Autodesk Inventor part; units mm, degrees
ref_plane "YZ Plane" through (0, 0, 0) normal (1, 0, 0) x (0, 1, 0)
ref_plane "XZ Plane" through (0, 0, 0) normal (0, 1, 0) x (-1, 0, 0)
ref_plane "XY Plane" through (0, 0, 0) normal (0, 0, 1) x (1, 0, 0)
sketch "Boceto2" plane through (0, 0, 0) normal (0, 0, 1) x (1, 0, 0)
  line L0 (-105.6698, 187.1112) -> (110.1141, 187.1112) construction
  line L1 (110.1141, 187.1112) -> (110.1141, -25.0762) construction
  line L2 (110.1141, -25.0762) -> (-105.6698, -25.0762) construction
  line L3 (-105.6698, -25.0762) -> (-105.6698, 187.1112) construction
  line L4 (0, 0) -> (0, 52.867)
  line L5 (0, 52.867) -> (0, 0)
  line L6 (-43.8447, 1.5105) -> (-43.8447, 13.5944)
  line L7 (-43.8447, 13.5944) -> (-37.8028, 21.1468)
  line L8 (-37.8028, 21.1468) -> (-39.3133, 27.944)
  line L9 (-39.3133, 27.944) -> (-36.2923, 36.2517)
  line L10 (-36.2923, 36.2517) -> (-32.6671, 40.7831)
  line L11 (-32.6671, 40.7831) -> (-30.2503, 43.8041)
  line L12 (-30.2503, 43.8041) -> (-27.2294, 47.5803)
  line L13 (-27.2294, 47.5803) -> (-27.2294, 52.867)
  line L14 (-27.2294, 52.867) -> (-23, 52.867)
  line L15 (0, 52.867) -> (-23, 52.867)
  line L16 (-27.2294, 52.867) -> (-23, 52.867)
  line L17 (0, 0) -> (-43.8447, 0)
  line L18 (-43.8447, 0) -> (-43.8447, 1.5105)
  dimension "d18" = 23
revolve "Revolución1" add sketch "Boceto2" angle 360 about axis through (0, 0, 0) along (0, 1, 0)
properties part number "KINGHT BASE 1.1"
Can you work these out from the model? Positions are in its coordinate system, mm. A direction names the side the tool comes from. Give positions to 0.01 mm unless a question says otherwise; leave off trailing zeros. Loops run counter-clockwise (first coordinate to the right, second up) from the corner with the lowest first, then second, coordinate; pieces in that order, holes last. Notation, with made-up numbers: M -17.5,63.25 L 23.5,63.25 A21 cw 23.5,69.25 Z; hole C 80,52 d4. An arc over 180 degrees is marked long. One line per item, written item: value. Start each with the question number.
1) If we section it at A-A, the plane x = 0: Write out the boundary of the cut face in (y, z).
2) Thinking about a two-plate mould opening in Y: for faces 1 (the face through (1, 0, 1)), 2 (the face through (0, 52.867, 0)), 3 (the face through (8.277, 20.674, 37.273)), 4 (the face through (8.215, 21.572, -36.996)), which applies, +Y half, -Y half, draft (parallel to the pull), parting line (faces both ways), or undercut?
3) If I drill on line 1 (Y direction, x = 3.5, z = -32.5); line 2 (X direction, y = 20.5, z = 9.5); line 3 (Y direction, x = 13.5, z = 31.5), over which ranges is the centre line in solid material (lowest first)? Write a range as [from, to].
4) If we section it at C-C, the plane z = 0: Write out the boundary of the cut face in (x, y), and give its area (3 significant figures).
5) If we section it at B-B, the plane y = 11: Write out the boundary of the cut face in (x, z), and give its area (3 significant figures).
6) If we section it at D-D, the plane y = 16.5: Write out the boundary of the cut face in (x, z).
7) On a 3-axis mill with a long thin cutter (end or side, diameter ignored), from which of +Z, -Z, +X, -X, +Y, -Y can I reach the whole of each face in a straight line? I mean faces 5 (the face through (5.903, 50.261, -26.582)), 6 (the face through (-41.82, 6.89, 13.17)). Say none if no direction works.
8) I'm going to push flat-ended pins straight in: pin 1 (2 mm diameter, centred on x = 21.5, y = 11.5, fed in from -Z); pin 2 (6 mm diameter, centred on y = 12.5, z = 6.5, fed in from -X); pin 3 (3 mm diameter, centred on x = -27, z = -33, fed in from +Y). Where does each tip first touch, or does it pass through?
Completed:
1. outline: M 0,-43.84 L 13.59,-43.84 L 21.15,-37.8 L 27.94,-39.31 L 36.25,-36.29 L 40.78,-32.67 L 43.8,-30.25 L 47.58,-27.23 L 52.87,-27.23 L 52.87,27.23 L 47.58,27.23 L 43.8,30.25 L 40.78,32.67 L 36.25,36.29 L 27.94,39.31 L 21.15,37.8 L 13.59,43.84 L 0,43.84 Z
2. face 1: -Y half
2. face 2: +Y half
2. face 3: undercut
2. face 4: undercut
3. line 1: y = [0, 40.76]
3. line 2: x = [-37.12, 37.12]
3. line 3: y = [0, 38.78]
4. outline: M -43.84,0 L 43.84,0 L 43.84,13.59 L 37.8,21.15 L 39.31,27.94 L 36.29,36.25 L 32.67,40.78 L 30.25,43.8 L 27.23,47.58 L 27.23,52.87 L -27.23,52.87 L -27.23,47.58 L -30.25,43.8 L -32.67,40.78 L -36.29,36.25 L -39.31,27.94 L -37.8,21.15 L -43.84,13.59 Z
4. area: 3,970 mm^2
5. outline: C 0,0 d87.69
5. area: 6,040 mm^2
6. outline: C 0,0 d83.04
7. face 5: +Y
7. face 6: +Y, -Y
8. pin 1: stops at z = -38.76
8. pin 2: stops at x = -43.7
8. pin 3: stops at y = 16.98
